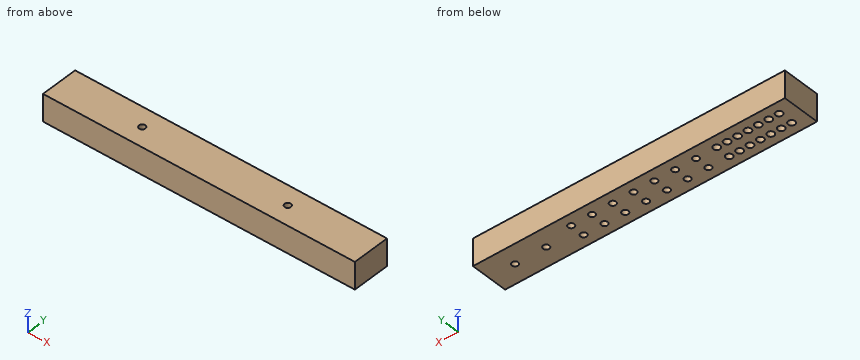
from build123d import *

# Parameters (mm, degrees)
SKETCH_W                 = 300
SKETCH_H                 = 36
PAD_DEPTH                = 26
SKETCH001_R              = 3
SKETCH001_R_2            = 1.6
POCKET_DEPTH             = 20
SKETCH002_R              = 3
POCKET001_DEPTH          = 15
SKETCH003_R              = 3.25
POCKET002_DEPTH          = 7
CLONE002_PLACEMENT_ANGLE = 180


with BuildPart() as part:
    # Sketch → Pad (new body)
    with BuildSketch(Plane.XY):
        with Locations((150, 18)):
            Rectangle(SKETCH_W, SKETCH_H)
    extrude(amount=-PAD_DEPTH)

    # Sketch001 (on Face5 of Pad) → Pocket (cut)
    with BuildSketch(Plane.XY):
        with Locations((25, 18)):
            Circle(SKETCH001_R)
        with Locations((55, 18)):
            Circle(SKETCH001_R)
        with Locations((85, 25)):
            Circle(SKETCH001_R)
        with Locations((105, 25)):
            Circle(SKETCH001_R)
        with Locations((125, 25)):
            Circle(SKETCH001_R)
        with Locations((145, 25)):
            Circle(SKETCH001_R)
        with Locations((165, 25)):
            Circle(SKETCH001_R)
        with Locations((185, 25)):
            Circle(SKETCH001_R)
        with Locations((205, 25)):
            Circle(SKETCH001_R)
        with Locations((225, 25)):
            Circle(SKETCH001_R_2)
        with Locations((235, 25)):
            Circle(SKETCH001_R_2)
        with Locations((245, 25)):
            Circle(SKETCH001_R_2)
        with Locations((255, 25)):
            Circle(SKETCH001_R_2)
        with Locations((265, 25)):
            Circle(SKETCH001_R_2)
        with Locations((275, 25)):
            Circle(SKETCH001_R_2)
        with Locations((285, 25)):
            Circle(SKETCH001_R_2)
        with Locations((85, 11)):
            Circle(SKETCH001_R)
        with Locations((105, 11)):
            Circle(SKETCH001_R)
        with Locations((125, 11)):
            Circle(SKETCH001_R)
        with Locations((145, 11)):
            Circle(SKETCH001_R)
        with Locations((165, 11)):
            Circle(SKETCH001_R)
        with Locations((185, 11)):
            Circle(SKETCH001_R)
        with Locations((205, 11)):
            Circle(SKETCH001_R)
        with Locations((235, 11)):
            Circle(SKETCH001_R_2)
        with Locations((245, 11)):
            Circle(SKETCH001_R_2)
        with Locations((255, 11)):
            Circle(SKETCH001_R_2)
        with Locations((265, 11)):
            Circle(SKETCH001_R_2)
        with Locations((275, 11)):
            Circle(SKETCH001_R_2)
        with Locations((285, 11)):
            Circle(SKETCH001_R_2)
        with Locations((225, 11)):
            Circle(SKETCH001_R_2)
    extrude(amount=-POCKET_DEPTH, mode=Mode.SUBTRACT)

    # Sketch002 (on Face5 of Pocket) → Pocket001 (cut)
    with BuildSketch(Plane(origin=(0, 0, -26), x_dir=(1, 0, 0), z_dir=(0, 0, -1))):
        with Locations((80, -18)):
            Circle(SKETCH002_R)
        with Locations((220, -18)):
            Circle(SKETCH002_R)
    extrude(amount=-POCKET001_DEPTH, mode=Mode.SUBTRACT)

    # Sketch003 (on Face4 of Pocket) → Pocket002 (cut)
    with BuildSketch(Plane.XY):
        with Locations((225, 11)):
            Circle(SKETCH003_R)
        with Locations((235, 11)):
            Circle(SKETCH003_R)
        with Locations((245, 11)):
            Circle(SKETCH003_R)
        with Locations((255, 11)):
            Circle(SKETCH003_R)
        with Locations((265, 11)):
            Circle(SKETCH003_R)
        with Locations((275, 11)):
            Circle(SKETCH003_R)
        with Locations((285, 11)):
            Circle(SKETCH003_R)
        with Locations((225, 25)):
            Circle(SKETCH003_R)
        with Locations((235, 25)):
            Circle(SKETCH003_R)
        with Locations((245, 25)):
            Circle(SKETCH003_R)
        with Locations((255, 25)):
            Circle(SKETCH003_R)
        with Locations((265, 25)):
            Circle(SKETCH003_R)
        with Locations((275, 25)):
            Circle(SKETCH003_R)
        with Locations((285, 25)):
            Circle(SKETCH003_R)
    extrude(amount=-POCKET002_DEPTH, mode=Mode.SUBTRACT)


with BuildPart() as part_1:
    # Clone002 placement: moved
    add(part.part.moved(Location((300, 0, -26))).rotate(Axis((300, 0, -26), (0, 1, 0)), CLONE002_PLACEMENT_ANGLE))


solid = part_1.part
Verification items for the finished model (mm, model axes). Coordinates: 2 decimals unless noted, no trailing zeros. Write each loop counter-clockwise with the first axis right and the second up, starting at its lowest first coordinate (ties: lowest second). Pieces come first, ordered by that corner, then holes. Notation, with made-up numbers: (-26.75, -39) -> (-12.75, -39) arc R23 ccw to (-12.75, -22) -> close; hole circle Ø6 at (55, 68.25). An arc over 180 degrees is marked (long way). One line per item, written item: value. Start each with the question number.
Q1. Go/stop test with flat-tipped pins: P1, Ø1, axis at x = 25, y = 10.5, coming from the -Z side; P2, Ø4, axis at x = 25, y = 25, coming from the -Z side. Record where each tip stops, or that it passes through.
Q2. Cross-section at B-B on y = 18. Enter the section's corners in (x, z).
Q3. Cross-section at C-C on x = 175. Enter the section's corners in (y, z), and give its area (3 significant figures).
Q4. Cross-section at A-A on z = -21.75. State how many separate pieces and enclosed holes the cut face has, and give its area (3 significant figures).
Q5. Thickness scan on L1, parallel to Y at x = 115, z = -13.75; L2, parallel to Y at x = 25, z = -23.25; L3, parallel to Y at x = 80.5, z = -12. Record the ranges inside material, lowest first. Write a range as from..to.
Checked values:
1. P1: stops at z = -6
1. P2: stops at z = -19
2. outline: (0, -26) -> (242, -26) -> (242, -6) -> (248, -6) -> (248, -26) -> (272, -26) -> (272, -6) -> (278, -6) -> (278, -26) -> (300, -26) -> (300, 0) -> (223, 0) -> (223, -15) -> (217, -15) -> (217, 0) -> (83, 0) -> (83, -15) -> (77, -15) -> (77, 0) -> (0, 0) -> close
3. outline: (0, -26) -> (8, -26) -> (8, -6) -> (14, -6) -> (14, -26) -> (22, -26) -> (22, -6) -> (28, -6) -> (28, -26) -> (36, -26) -> (36, 0) -> (0, 0) -> close
3. area: 696 mm²
4. separate pieces: 1
4. enclosed holes: 30
4. area: 9,880 mm²
5. L1: y = 0..8, 14..22, 28..36
5. L2: y = 0..7.75, 14.25..21.75, 28.25..36
5. L3: y = 0..15.04, 20.96..36
